Here's how the part is built. I have some questions about the finished solid (model axes, mm). Face numbers are marked on the shaded views. A direction names the side the tool comes from. Give positions to 0.01 mm unless a question says otherwise; leave off trailing zeros. Write each loop counter-clockwise with the first axis right and the second up, starting at its lowest first coordinate (ties: lowest second). Pieces come first, ordered by that corner, then holes. Notation, with made-up numbers: (57.5, 63.5) -> (88.5, 63.5) arc R3 ccw to (88.5, 68.5) -> close; hole circle Ø3 at (48.5, -21). An arc over 180 degrees is marked (long way). Return JSON: item names as keys, results as strings.
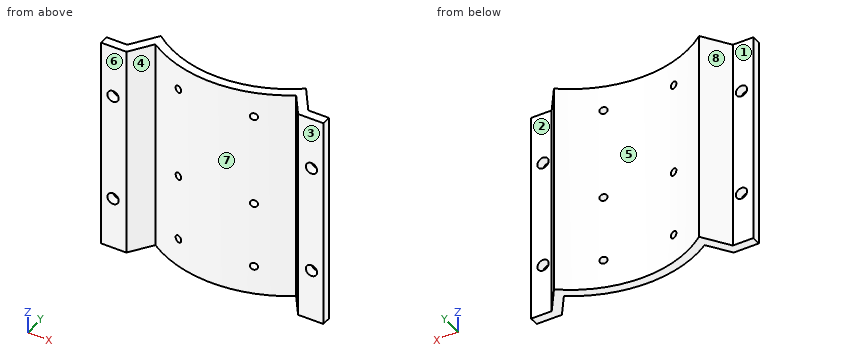
from build123d import *

# Parameters (mm, degrees)
BOSS_EXTRUDE1_DEPTH         = 149.606
SKETCH5_R                   = 2.54
CUT_EXTRUDE1_DEPTH          = 25.4
SKETCH4_R                   = 2.54
CUT_EXTRUDE2_DEPTH          = 25.4
TAP_DRILL_FOR_3_8_16_TAP1_D = 7.9375


with BuildPart() as part:
    # Sketch1 → Boss-Extrude1 (new body)
    with BuildSketch(Plane.XY):
        Polygon((78.143354, 6.951268616), (63.668954771, 6.951268616), (65.564969481, 4.243478987), (60.363354, 0.601268616), (78.143354, 0.601268616), align=None)
        with BuildLine():
            Line((-50.996127998, 25.049940912), (-63.668954771, 6.951268616))
            Line((-63.668954771, 6.951268616), (-60.363354, 6.951268616))
            Line((-60.363354, 6.951268616), (-60.363354, 0.601268616))
            Line((-60.363354, 0.601268616), (-49.49782024, 16.118858997))
            ThreePointArc((-49.49782024, 16.118858997), (0, 1.06448034), (49.49782024, 16.118858997))
            Line((49.49782024, 16.118858997), (60.363354, 0.601268616))
            Line((60.363354, 0.601268616), (60.363354, 6.951268616))
            Line((60.363354, 6.951268616), (63.668954771, 6.951268616))
            Line((63.668954771, 6.951268616), (50.996127998, 25.049940912))
            ThreePointArc((50.996127998, 25.049940912), (0, 7.41448034), (-50.996127998, 25.049940912))
        make_face()
        Polygon((65.564969481, 4.243478987), (63.668954771, 6.951268616), (60.363354, 6.951268616), (60.363354, 0.601268616), align=None)
        Polygon((-63.668954771, 6.951268616), (-78.143354, 6.951268616), (-78.143354, 0.601268616), (-60.363354, 0.601268616), (-65.564969481, 4.243478987), align=None)
        Polygon((-60.363354, 6.951268616), (-63.668954771, 6.951268616), (-65.564969481, 4.243478987), (-60.363354, 0.601268616), align=None)
    extrude(amount=BOSS_EXTRUDE1_DEPTH)

    # Sketch5 → Cut-Extrude1 (cut)
    with BuildSketch(Plane(origin=(0.999392331, 3.192633299, 0), x_dir=(0.9543356688296087, -0.29873639081896847, 0), z_dir=(0.29873639081896847, 0.9543356688296087, 0))):
        with Locations(Location((-26.875664159, -20.32, 0), (0, 0, 180))):
            Circle(SKETCH5_R)
        with Locations(Location((-26.875664159, -67.056, 0), (0, 0, 180))):
            Circle(SKETCH5_R)
        with Locations(Location((-26.875664159, -131.826, 0), (0, 0, 180))):
            Circle(SKETCH5_R)
    extrude(amount=-CUT_EXTRUDE1_DEPTH, mode=Mode.SUBTRACT)

    # Sketch4 → Cut-Extrude2 (cut)
    with BuildSketch(Plane(origin=(-0.999392331, 3.192633299, 0), x_dir=(-0.9543356688296079, -0.2987363908189716, 0), z_dir=(0.2987363908189716, -0.9543356688296079, 0))):
        with Locations((-26.875664159, -131.826)):
            Circle(SKETCH4_R)
        with Locations((-26.875664159, -67.056)):
            Circle(SKETCH4_R)
        with Locations((-26.875664159, -20.32)):
            Circle(SKETCH4_R)
    extrude(amount=CUT_EXTRUDE2_DEPTH, mode=Mode.SUBTRACT)

    # Tap Drill for 3_8-16 Tap1 (through all)
    with Locations(Plane(origin=(0, 6.951268616, 0), x_dir=(1, 0, 0), z_dir=(0, 1, 0))):
        with Locations((-69.761354, -112.776), (-69.761354, -36.576), (69.761354, -112.776), (69.761354, -36.576)):
            Hole(TAP_DRILL_FOR_3_8_16_TAP1_D / 2)


solid = part.part
1. Suppose I cut it at B-B, the plane z = 84.5. List the corners of the cut face in (x, y) for me, and give its area (3 significant figures).
Taken from the geometry:
{"outline": "(-78.14, 0.6) -> (-60.36, 0.6) -> (-49.5, 16.12) arc R88.9 ccw to (49.5, 16.12) -> (60.36, 0.6) -> (78.14, 0.6) -> (78.14, 6.95) -> (63.67, 6.95) -> (51, 25.05) arc R82.55 cw to (-51, 25.05) -> (-63.67, 6.95) -> (-78.14, 6.95) -> close", "area": "1,150 mm²"}
2. Suppose I cut it at D-D, the plane x = -54.5. List the corners of the cut face in (y, z) for me (3 decimals), and give its area (3 significant figures).
Taken from the geometry:
{"outline": "(8.975, 0) -> (20.046, 0) -> (20.046, 149.606) -> (8.975, 149.606) -> close", "area": "1,660 mm²"}
3. Which directions (+Z, -Z, +X, -X, +Y, -Y) give clear straight access to the entire face, cutting with the end or side of a thin tool? Please do the marked faces 1, 2, 3 and 4.
Taken from the geometry:
{"face 1": "+Z, -Z, -X, +Y", "face 2": "+Z, -Z, +X, +Y", "face 3": "+Z, -Z, +X, -X, -Y", "face 4": "+Z, -Z, -Y"}
4. If we mould it in two halves opening along X, with no side actions, what happens to the marked faces 5, 6, 7 and 8? For each: released by +X, released by -X, zero draft, split by the parting line, or undercut.
Taken from the geometry:
{"face 5": "undercut", "face 6": "zero draft", "face 7": "undercut", "face 8": "released by -X"}
5. If I drill on line 1 (X direction, y = 14.75, z = 104.5); line 2 (X direction, y = 20.75, z = 85.5); line 3 (Y direction, x = 67.5, z = 24), over which ranges is the centre line in solid material (lowest first)? Write a range as [from, to].
Taken from the geometry:
{"line 1": "x = [-58.21, -50.46], [-47.39, -34.02], [34.02, 47.39], [50.46, 58.21]", "line 2": "x = [-54.01, -44.99], [44.99, 54.01]", "line 3": "y = [0.6, 6.95]"}
6. Suppose I cut it at A-A, the plane y = 19.75. List the corners of the cut face in (x, z) for me.
Taken from the geometry:
{"outline": "(-54.71, 0) -> (-43.41, 0) -> (-43.41, 149.61) -> (-54.71, 149.61) -> close; (43.41, 0) -> (54.71, 0) -> (54.71, 149.61) -> (43.41, 149.61) -> close"}
7. For pin 1 Ø5 at (x, z) = (-69.76, 112.78) entering from -Y; pin 2 Ø4 at (x, z) = (8, 127) entering from +Y; pin 3 Ø12 at (x, z) = (35.5, 108) entering from +Y; pin 4 Ø16 at (x, z) = (73.5, 90) entering from +Y, each with a flat end and sliding along its axis, tell me the tip position at first contact or that it passes through.
Taken from the geometry:
{"pin 1": "passes through", "pin 2": "stops at y = 8.02", "pin 3": "stops at y = 18.6", "pin 4": "stops at y = 6.95"}
8. Suppose I cut it at C-C, the plane x = 4.5. List the corners of the cut face in (y, z) for me, and give its area (3 significant figures).
Taken from the geometry:
{"outline": "(1.18, 0) -> (7.54, 0) -> (7.54, 149.61) -> (1.18, 149.61) -> close", "area": "951 mm²"}
